Design review of the part built by this model. Coordinates are the model's own, in mm. A direction names the side the tool comes from. Coordinates: 2 decimals unless noted, no trailing zeros. Write each loop counter-clockwise with the first axis right and the second up, starting at its lowest first coordinate (ties: lowest second). Pieces come first, ordered by that corner, then holes. Notation, with made-up numbers: (22.5, -28.75) -> (42.5, -28.75) arc R19 ccw to (42.5, -3.75) -> close; hole circle Ø6 at (62.5, 18.25). An arc over 180 degrees is marked (long way). One line per question, with ' | ' between items. Start each with the question number.
Q1. Add section B-B on z = 81.5. State the section outline as (x, y) points, and give its area (3 significant figures).
Q2. For P1, Ø4, axis at y = -66.5, z = 81, coming from the +X side; P2, Ø22, axis at x = -89.5, y = -1, coming from the +Z side; P3, Ø18, axis at x = -91, y = 2, coming from the -Z side, all flat-tipped, find the tip position at first contact; note any pin that passes through.
Q3. Add section C-C on x = 80.5. State the section outline as (y, z) points.
Q4. Draft analysis for pull direction Z (two halves, no side actions). For faces 1 (the cylindrical face through (-103.963, 11.993, -0.799)), 2 (the flat face through (-55, -15, 0)), 3 (the cylindrical face through (-2.253, -79.93, 68.795)), 4 (the cylindrical face through (-64.1, 0.73, 19.04)), state which applies: pulls with the +Z half, pulls with the -Z half, needs draft (parallel to the pull), parting line crosses it, or undercut.
Q5. For faces 5 (the flat face through (54, -15, 0)), 6 (the flat face through (-0.21, -26.967, 15.373)), 7 (the cylindrical face through (-66.286, 0.142, 8.324)), list the 3-axis set-ups (+Z, -Z, +X, -X, +Y, -Y) from which the entire face can be reached by the end or side of a thin tool; tool diameter is ignored.
Q6. Wall thickness on probe 1 along Y at (x, z) = (-31, 1.6); probe 2 along Z at (x, y) = (46.5, 14); probe 3 along Y at (x, z) = (73, -1.5): over which ranges is each line inside the solid? List them lowest first.
from build123d import *

# Parameters (mm, degrees)
IZIM1_W                     = 218
IZIM1_H                     = 30
Y_KSEKLIK_EKSTR_ZYON1_DEPTH = 5
RADYUS1_R                   = 20
IZIM3_R                     = 10
KES_EKSTR_ZYON1_DEPTH       = 4
PAH1_SIZE                   = 3
IZIM5_R                     = 5
KES_EKSTR_ZYON3_DEPTH       = 119.749210232
Y_KSEKLIK_EKSTR_ZYON2_DEPTH = 20
IZIM9_W                     = 30
IZIM9_H                     = 21.4
Y_KSEKLIK_EKSTR_ZYON3_DEPTH = 3
IZIM9_3_W                   = 30
IZIM9_3_H                   = 21.4
KES_EKSTR_ZYON4_DEPTH       = 3
KES_EKSTR_ZYON5_DEPTH       = 40
RADYUS2_R                   = 10
RADYUS2_OF_AYNALAMA1_R      = 10


with BuildPart() as part:
    # Çizim1 → Yükseklik-Ekstrüzyon1 (new, symmetric)
    with BuildSketch(Plane.XY):
        Rectangle(IZIM1_W, IZIM1_H)
    extrude(amount=Y_KSEKLIK_EKSTR_ZYON1_DEPTH, both=True)

    # Radyus1
    radyus1_edges = [part.edges().sort_by_distance(p)[0] for p in [
        (109, -15, 0),
        (-109, -15, 0),
    ]]
    fillet(radyus1_edges, radius=RADYUS1_R)

    # Çizim3 → Kes-Ekstrüzyon1 (cut)
    with BuildSketch(Plane.XY.offset(5)):
        with Locations((-91, 2)):
            Circle(IZIM3_R)
        with Locations((-31, 2)):
            Circle(IZIM3_R)
    extrude(amount=-KES_EKSTR_ZYON1_DEPTH, mode=Mode.SUBTRACT)

    # Pah1
    pah1_edges = [part.edges().sort_by_distance(p)[0] for p in [
        (-101, 2, 5),
        (-41, 2, 5),
    ]]
    chamfer(pah1_edges, length=PAH1_SIZE - 0.0001)  # a hair under: the kernel refuses the full size

    # Çizim4 → Döndür1 (revolve)
    with BuildSketch(Plane(origin=(-61.85, 0, 0), x_dir=(0, 0, -1), z_dir=(1, 0, 0)), mode=Mode.PRIVATE) as d_nd_r1_sk:
        Polygon((-20.498711306, 18.495190528), (-24.248711306, 12), (10.392304845, -8), (14.142304845, -1.504809472), align=None)
    revolve(d_nd_r1_sk.sketch.rotate(Axis((-61.85, 12, 24.248711306), (0, -0.49999999999999767, -0.86602540378444)), 180), axis=Axis((-61.85, 12, 24.248711306), (0, -0.49999999999999767, -0.86602540378444)))

    # Çizim5 → Kes-Ekstrüzyon3 (cut, through all)
    with BuildSketch(Plane(origin=(0, 13.5, 23.382685902), x_dir=(1, 0, 0), z_dir=(0, 0.4999999999999978, 0.86602540378444))):
        with Locations(Location((-61.85, -1.732050808, 0), (0, 0, 270))):
            Circle(IZIM5_R)
    extrude(amount=-KES_EKSTR_ZYON3_DEPTH, mode=Mode.SUBTRACT)

    # Çizim7 → Yükseklik-Ekstrüzyon2 (add, symmetric)
    with BuildSketch(Plane(origin=(0, 0, 0), x_dir=(0, 0, -1), z_dir=(1, 0, 0))):
        Polygon((5, -15), (-5, -15), (-33.867513459, -65), (-91.641016151, -65), (-91.641016151, -75), (-29.641016151, -75), align=None)
    extrude(amount=Y_KSEKLIK_EKSTR_ZYON2_DEPTH, both=True)

    # Çizim9 → Yükseklik-Ekstrüzyon3 (add)
    with BuildSketch(Plane(origin=(0, -1.584936491, -2.745190528), x_dir=(1, 0, 0), z_dir=(0, 0.4999999999999977, 0.86602540378444))):
        with Locations((0, -31.190381057)):
            Rectangle(IZIM9_W, IZIM9_H)
    extrude(amount=Y_KSEKLIK_EKSTR_ZYON3_DEPTH)

    # Çizim9<3> → Kes-Ekstrüzyon4 (cut)
    with BuildSketch(Plane(origin=(0, -1.584936491, -2.745190528), x_dir=(1, 0, 0), z_dir=(0, 0.4999999999999977, 0.86602540378444))):
        with Locations((0, -57.525407976)):
            Rectangle(IZIM9_3_W, IZIM9_3_H)
    extrude(amount=-KES_EKSTR_ZYON4_DEPTH, mode=Mode.SUBTRACT)

    # Çizim11 → Döndür2 (revolve)
    with BuildSketch(Plane(origin=(0, 0, 0), x_dir=(0, 0, -1), z_dir=(1, 0, 0)), mode=Mode.PRIVATE) as d_nd_r2_sk:
        with BuildLine():
            Line((-61.641016151, -23.147719704), (-61.641016151, -85))
            Line((-61.641016151, -85), (-54.141016151, -85))
            Line((-54.141016151, -85), (-54.141016151, -75))
            Line((-54.141016151, -75), (-56.641016151, -75))
            Line((-56.641016151, -75), (-56.641016151, -63))
            ThreePointArc((-56.641016151, -63), (-57.519695808, -60.878679656), (-59.641016151, -60))
            Line((-59.641016151, -60), (-59.641016151, -36.252262247))
            ThreePointArc((-59.641016151, -36.252262247), (-55.765967633, -28.955966756), (-61.641016151, -23.147719704))
        make_face()
    revolve(d_nd_r2_sk.sketch.rotate(Axis((0, -23.147719704, 61.641016151), (0, -1, 0)), 180), axis=Axis((0, -23.147719704, 61.641016151), (0, -1, 0)))

    # Çizim12 → Kes-Ekstrüzyon5 (cut)
    with BuildSketch(Plane(origin=(0, 15, 0), x_dir=(1, 0, 0), z_dir=(0, 1, 0))):
        Polygon((-109, 5), (-109, -5), (-105.52, 5), align=None)
    kes_ekstr_zyon5 = extrude(amount=-KES_EKSTR_ZYON5_DEPTH, mode=Mode.SUBTRACT)

    # Radyus2
    radyus2_edges = [part.edges().sort_by_distance(p)[0] for p in [
        (-107.26, 15, 0),
    ]]
    fillet(radyus2_edges, radius=RADYUS2_R)

    # Aynalama1: Kes-Ekstrüzyon5 across plane
    add(kes_ekstr_zyon5.mirror(Plane(origin=(0, 0, 0), x_dir=(0, 0, 1), z_dir=(1, 0, 0))), mode=Mode.SUBTRACT)

    # Radyus2 of Aynalama1
    radyus2_of_aynalama1_edges = [part.edges().sort_by_distance(p)[0] for p in [
        (107.26, 15, 0),
    ]]
    fillet(radyus2_of_aynalama1_edges, radius=RADYUS2_OF_AYNALAMA1_R)


solid = part.part
Output values:
1) outline: (-20, -75) -> (20, -75) -> (20, -65) -> (-20, -65) -> close | area: 400 mm2
2) P1: stops at x = 20 | P2: stops at z = 5 | P3: stops at z = -5
3) outline: (-15, -5) -> (15, -5) -> (15, 5) -> (-15, 5) -> close
4) face 1: pulls with the -Z half | face 2: needs draft | face 3: parting line crosses it | face 4: undercut
5) face 5: +Z, -Z, +X, -Y | face 6: +X, -X, +Y | face 7: none
6) probe 1: y = -15 to -8, 12 to 15 | probe 2: z = -5 to 5 | probe 3: y = -15 to 15
